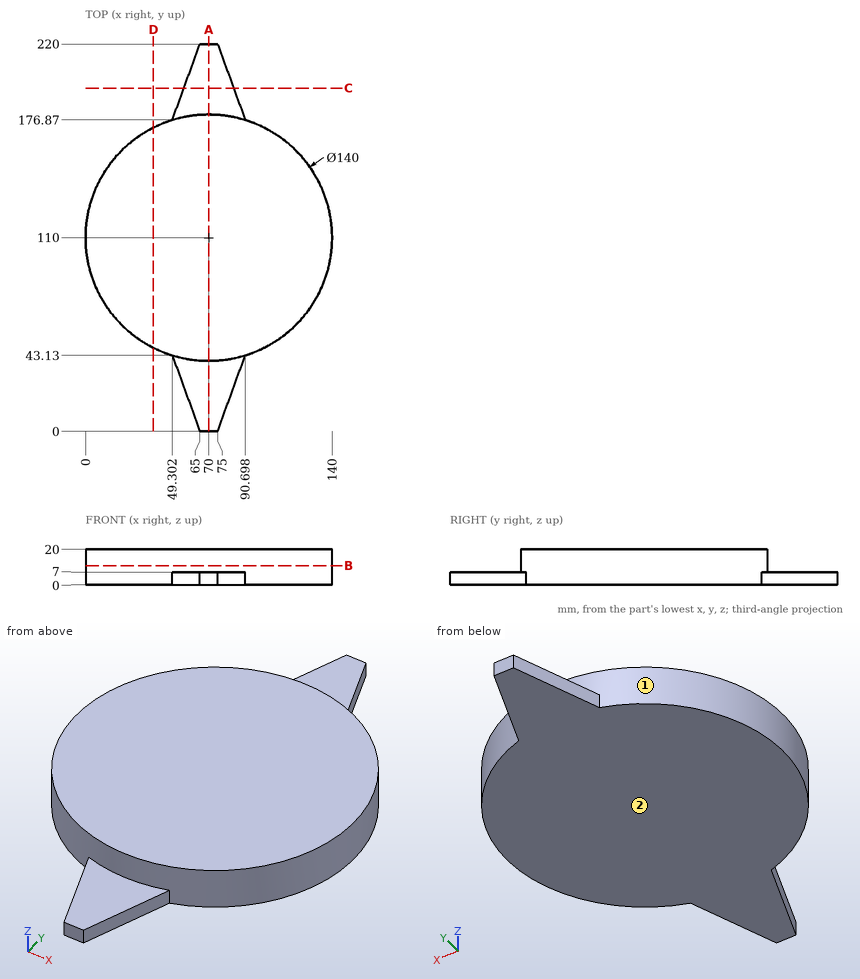
Input: dimensioned drawing with shaded views. Units: mm. Origin: part minimum x, y, z. A direction names the side the tool comes from. Coordinates: 2 decimals unless noted, no trailing zeros. Order: outer loops, then holes, each group sorted by start corner. A loop starts at its lowest first (then second) coordinate and runs counter-clockwise, first axis right, second up. Notation, with made-up numbers: M 61.5,39.25 L 118.5,39.25 A20 cw 118.5,67.25 Z; hole C 33,74.25 d9. An arc over 180 degrees is marked long. Write each question's results on one line, items separated by ' | '. Start each with the question number.
Item 1: Cut plane C-C (y = 195). Return loops of the section in (x, z), and give its area (3 significant figures).
Item 2: First-contact query: pin 1 Ø6 at (x, z) = (56.5, 11.5) entering from +Y; pin 2 Ø4 at (y, z) = (159, 2.5) entering from -X (1 decimal); pin 3 Ø20.5 at (x, y) = (65.5, 206) entering from +Z; pin 4 Ø12 at (y, z) = (187, 17) entering from -X. Flat tips, straight axial feed; report the tip coordinate or a pass-through.
Item 3: Cut plane B-B (z = 10.75). Return loops of the section in (x, y).
Item 4: Cut plane A-A (x = 70). Return loops of the section in (y, z), and give its area (3 significant figures).
Item 5: Line query: probe 1 along Z at (x, y) = (60.5, 180.5); probe 2 along Y at (x, z) = (30, 19); probe 3 along Y at (x, z) = (49, 4). Output: solid intervals per line, ascending.
Item 6: Set-up query: the marked faces 1 and 2. Return all of +Z, -Z, +X, -X, +Y, -Y with unobstructed straight access to the full face (end or side cutting, diameter ignored); none if empty.
Item 7: Cut plane D-D (x = 38.5). Return loops of the section in (y, z).
Checked values:
1) outline: M 55.9,0 L 84.1,0 L 84.1,7 L 55.9,7 Z | area: 197 mm2
2) pin 1: stops at y = 179.21 | pin 2: stops at x = 18.1 | pin 3: stops at z = 7 | pin 4: passes through
3) outline: C 70,110 d140
4) outline: M 0,0 L 220,0 L 220,7 L 180,7 L 180,20 L 40,20 L 40,7 L 0,7 Z | area: 3,360 mm2
5) probe 1: z = 0 to 7 | probe 2: y = 52.55 to 167.45 | probe 3: y = 43.22 to 176.78
6) face 1: +Z | face 2: -Z, +X, -X, +Y, -Y
7) outline: M 47.49,0 L 172.51,0 L 172.51,20 L 47.49,20 Z
